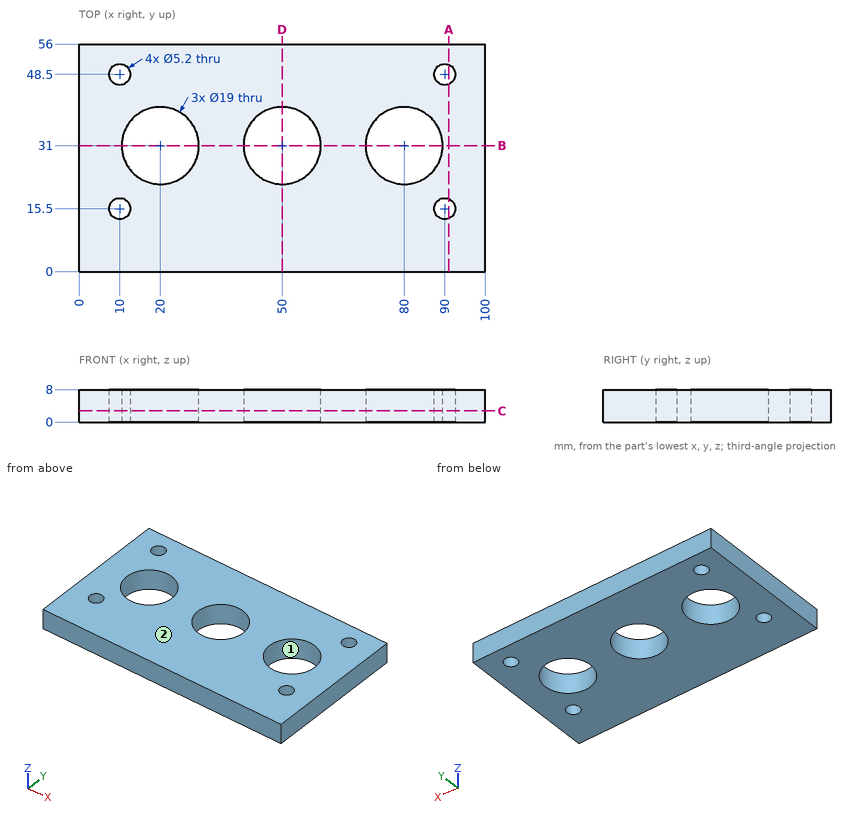
Check sheet for the drawn part. Datum: minimum x, y, z corner. Units: mm. Give positions to 0.01 mm unless a question says otherwise; leave off trailing zeros. Order: outer loops, then holes, each group sorted by start corner. A loop starts at its lowest first (then second) coordinate and runs counter-clockwise, first axis right, second up. Notation, with made-up numbers: (39, 30) -> (82, 30) arc R17 cw to (82, 57) -> close; hole circle Ø7 at (-14.75, 60.25). An arc over 180 degrees is marked (long way). Use a Markdown table: item, result.
1) Section check B-B, the plane y = 31. Record the boundary of the cut face in (x, z).
Results:
| item | result |
|---|---|
| outline | (0, 0) -> (10.5, 0) -> (10.5, 8) -> (0, 8) -> close; (29.5, 0) -> (40.5, 0) -> (40.5, 8) -> (29.5, 8) -> close; (59.5, 0) -> (70.5, 0) -> (70.5, 8) -> (59.5, 8) -> close; (89.5, 0) -> (100, 0) -> (100, 8) -> (89.5, 8) -> close |
2) Section check A-A, the plane x = 91. Record the boundary of the cut face in (y, z).
Results:
| item | result |
|---|---|
| outline | (0, 0) -> (13.1, 0) -> (13.1, 8) -> (0, 8) -> close; (17.9, 0) -> (46.1, 0) -> (46.1, 8) -> (17.9, 8) -> close; (50.9, 0) -> (56, 0) -> (56, 8) -> (50.9, 8) -> close |
3) Section check C-C, the plane z = 2.75. Record the boundary of the cut face in (x, y).
Results:
| item | result |
|---|---|
| outline | (0, 0) -> (100, 0) -> (100, 56) -> (0, 56) -> close; hole circle Ø5.2 at (10, 15.5); hole circle Ø5.2 at (10, 48.5); hole circle Ø19 at (20, 31); hole circle Ø19 at (50, 31); hole circle Ø19 at (80, 31); hole circle Ø5.2 at (90, 15.5); hole circle Ø5.2 at (90, 48.5) |
4) Material ranges on probe 1 along Y at (x, z) = (20, 4.5); probe 2 along X at (y, z) = (33.5, 6); probe 3 along X at (y, z) = (17, 4.25), recorded low to high.
Results:
| item | result |
|---|---|
| probe 1 | 0 to 21.5, 40.5 to 56 |
| probe 2 | 0 to 10.83, 29.17 to 40.83, 59.17 to 70.83, 89.17 to 100 |
| probe 3 | 0 to 7.88, 12.12 to 87.88, 92.12 to 100 |
5) Mould release check, pull along X, two halves, no side actions. Record for the marked faces 1 and 2: pulls with the +X half, pulls with the -X half, needs draft (parallel to the pull), parting line crosses it, or undercut.
Results:
| item | result |
|---|---|
| face 1 | undercut |
| face 2 | needs draft |
6) Depth check by flat-ended pin: pin 1 Ø2 at (y, z) = (10.5, 7) entering from -X. Enter the tip coordinate at first touch or a pass-through.
Results:
| item | result |
|---|---|
| pin 1 | x = 0 |
7) Section check D-D, the plane x = 50. Record the boundary of the cut face in (y, z).
Results:
| item | result |
|---|---|
| outline | (0, 0) -> (21.5, 0) -> (21.5, 8) -> (0, 8) -> close; (40.5, 0) -> (56, 0) -> (56, 8) -> (40.5, 8) -> close |
